```python
from build123d import *

# Parameters (mm, degrees)
ESQUISSE1_W             = 30
ESQUISSE1_H             = 15
BOSS_EXTRU_1_DEPTH      = 10
ESQUISSE2_W             = 24
ESQUISSE2_H             = 9
ENL_V_MAT_EXTRU_1_DEPTH = 8
CONG_1_R                = 2
ESQUISSE3_R             = 1.75
ENL_V_MAT_EXTRU_2_DEPTH = 3
TROU_TARAUD_M31_D       = 2.5
TROU_TARAUD_M32_D       = 2.5


with BuildPart() as part:
    # Esquisse1 → Boss.-Extru.1 (new body)
    with BuildSketch(Plane.XY):
        Rectangle(ESQUISSE1_W, ESQUISSE1_H)
    extrude(amount=BOSS_EXTRU_1_DEPTH)

    # Esquisse2 → Enlèv. mat.-Extru.1 (cut)
    with BuildSketch(Plane(origin=(0, 0, 0), x_dir=(-1, 0, 0), z_dir=(0, 0, -1))):
        Rectangle(ESQUISSE2_W, ESQUISSE2_H)
    extrude(amount=-ENL_V_MAT_EXTRU_1_DEPTH, mode=Mode.SUBTRACT)

    # Congé1
    cong_1_edges = [part.edges().sort_by_distance(p)[0] for p in [
        (12, -4.5, 4),
        (12, 4.5, 4),
        (-12, 4.5, 4),
        (-12, -4.5, 4),
    ]]
    fillet(cong_1_edges, radius=CONG_1_R)

    # Esquisse3 → Enlèv. mat.-Extru.2 (cut, through all)
    with BuildSketch(Plane(origin=(0, 0, 8), x_dir=(-1, 0, 0), z_dir=(0, 0, -1))):
        Circle(ESQUISSE3_R)
    extrude(amount=-ENL_V_MAT_EXTRU_2_DEPTH, mode=Mode.SUBTRACT)

    # Trou taraudé M31 (through all)
    with Locations(Plane(origin=(0, -7.5, 0), x_dir=(-1, 0, 0), z_dir=(0, -1, 0))):
        with Locations((-10, -5)):
            Hole(TROU_TARAUD_M31_D / 2)

    # Trou taraudé M32 (through all)
    with Locations(Plane(origin=(0, -7.5, 0), x_dir=(-1, 0, 0), z_dir=(0, -1, 0))):
        with Locations((10, -5)):
            Hole(TROU_TARAUD_M32_D / 2)


solid = part.part
```
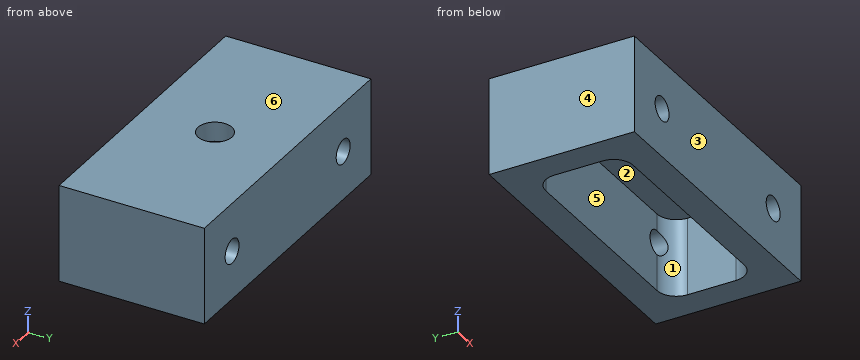
For this review, take the finished solid that the model builds, in its own axes (mm). Face numbers are marked on the shaded views. A direction names the side the tool comes from. Give positions to 0.01 mm unless a question says otherwise; leave off trailing zeros. Order: outer loops, then holes, each group sorted by start corner. A loop starts at its lowest first (then second) coordinate and runs counter-clockwise, first axis right, second up.
1) Take a section at B-B (x = 9.25). Give the boundary of the cut face in (y, z), then the cut area to 3 significant figures.
2) Insertion check: pin 1 (3 mm diameter, centred on x = 10, z = 5, fed in from -Y). The pin has a flat end and moves straight along its axis. Give the tip position at first contact, or say it passes through.
3) Wall thickness on line 1 (X direction, y = 6, z = 5); line 2 (X direction, y = -0.5, z = 6.75); line 3 (Y direction, x = -7.75, z = 2.5): over which ranges is each line inside the solid? List them lowest first.
4) For the marked faces 5 and 6, list the 3-axis set-ups (+Z, -Z, +X, -X, +Y, -Y) from which the entire face can be reached by the end or side of a thin tool; tool diameter is ignored.
5) Take a section at A-A (x = 0). Give the boundary of the cut face in (y, z).
6) Take a section at C-C (y = 5.5). Give the boundary of the cut face in (x, z).
7) Take a section at D-D (z = 7). Give the boundary of the cut face in (x, y), then the cut area to 3 significant figures.
8) The part is to be moulded in two halves that separate along Y. For the marked faces 1, 2, 3 and 4, say which applies: released by +Y, released by -Y, zero draft, split by the parting line, or undercut.
Derived:
1. outline: (-7.5, 0) - (-4.5, 0) - (-4.5, 4) - (-7.5, 4) - close; (-7.5, 6) - (-4.5, 6) - (-4.5, 8) - (4.5, 8) - (4.5, 6) - (7.5, 6) - (7.5, 10) - (-7.5, 10) - close; (4.5, 0) - (7.5, 0) - (7.5, 4) - (4.5, 4) - close
1. area: 66.0 mm2
2. pin 1: stops at y = -7.5
3. line 1: x = -15 to -11.25, -8.75 to 8.75, 11.25 to 15
3. line 2: x = -15 to -12, 12 to 15
3. line 3: y = -7.5 to -4.5, 4.5 to 7.5
4. face 5: -Z
4. face 6: +Z, +X, -X, +Y, -Y
5. outline: (-7.5, 0) - (-4.5, 0) - (-4.5, 8) - (-1.75, 8) - (-1.75, 10) - (-7.5, 10) - close; (1.75, 8) - (4.5, 8) - (4.5, 0) - (7.5, 0) - (7.5, 10) - (1.75, 10) - close
6. outline: (-15, 0) - (15, 0) - (15, 10) - (-15, 10) - close; hole circle Ø2.5 at (-10, 5); hole circle Ø2.5 at (10, 5)
7. outline: (-15, -7.5) - (15, -7.5) - (15, 7.5) - (-15, 7.5) - close; hole (-12, -2.5) arc R2 ccw to (-10, -4.5) - (10, -4.5) arc R2 ccw to (12, -2.5) - (12, 2.5) arc R2 ccw to (10, 4.5) - (-10, 4.5) arc R2 ccw to (-12, 2.5) - close
7. area: 237 mm2
8. face 1: undercut
8. face 2: undercut
8. face 3: released by -Y
8. face 4: zero draft
